```python
from build123d import *

# Parameters (mm, degrees)
BOSS_EXTRUDE2_DEPTH = 24.13
SKETCH3_W           = 24.13
SKETCH3_H           = 25.4
SKETCH3_R           = 8.89
CUT_EXTRUDE3_DEPTH  = 16.51
SKETCH4_W           = 138.37052371
SKETCH4_H           = 157.28988693
CUT_EXTRUDE4_DEPTH  = 8.89
CHAMFER1_SIZE       = 34.874144438
CHAMFER1_SIZE_2     = 10


with BuildPart() as part:
    # Sketch2 → Boss-Extrude2 (new body)
    # profile 1 of 2: a face of its own
    with BuildSketch(Plane(origin=(0, 0, 0), x_dir=(0, 0, -1), z_dir=(1, 0, 0))):
        Polygon((-111.06, -12.7), (-22.16, -12.7), (-22.16, 0), (-22.16, 12.7), (-111.06, 12.7), align=None)
    # profile 2 of 2: a face of its own
    with BuildSketch(Plane(origin=(0, 0, 0), x_dir=(0, 0, -1), z_dir=(1, 0, 0))):
        with BuildLine():
            Line((-22.16, -44.45), (-22.16, 44.45))
            ThreePointArc((-22.16, 44.45), (0, 66.61), (22.16, 44.45))
            Line((22.16, 44.45), (22.16, -44.45))
            ThreePointArc((22.16, -44.45), (0, -66.61), (-22.16, -44.45))
        make_face()
        with BuildLine():
            ThreePointArc((12, 44.45), (0, 56.45), (-12, 44.45))
            Line((-12, 44.45), (-12, -44.45))
            ThreePointArc((-12, -44.45), (0, -56.45), (12, -44.45))
            Line((12, -44.45), (12, 44.45))
        make_face(mode=Mode.SUBTRACT)
    extrude(amount=BOSS_EXTRUDE2_DEPTH)

    # Sketch3 → Cut-Extrude3 (cut)
    with BuildSketch(Plane.XY.offset(111.06)):
        with Locations((12.065, 0)):
            Rectangle(SKETCH3_W, SKETCH3_H)
        with Locations((10.4775, 0)):
            Circle(SKETCH3_R, mode=Mode.SUBTRACT)
    extrude(amount=-CUT_EXTRUDE3_DEPTH, mode=Mode.SUBTRACT)

    # Sketch4 → Cut-Extrude4 (cut)
    with BuildSketch(Plane.ZY):
        Rectangle(SKETCH4_W, SKETCH4_H)
    extrude(amount=-CUT_EXTRUDE4_DEPTH, mode=Mode.SUBTRACT)

    # Chamfer1
    # the kernel refuses this chamfer: 34.874144438, 10 mm, written as the material it adds along each edge
    with BuildSketch(Plane(origin=(8.89, 12.7, 69.185261855), x_dir=(0.010616657410321159, 0, -0.9999436417045873), z_dir=(0, -1, 0))) as chamfer1_piece_1_section:
        Polygon((CHAMFER1_SIZE * 0.999943641716, -CHAMFER1_SIZE * 0.0106166574104), (-CHAMFER1_SIZE_2 * 0.0106166574103, -CHAMFER1_SIZE_2 * 0.999943641705), (0, 0), align=None)
    chamfer1_piece_1 = extrude(amount=25.4, mode=Mode.PRIVATE)
    chamfer1_piece_1 = split(chamfer1_piece_1, bisect_by=Plane(origin=(0, 0, 56.832486902), z_dir=(1, 0, 0)), keep=Keep.TOP, mode=Mode.PRIVATE)
    add(chamfer1_piece_1)


solid = part.part
```
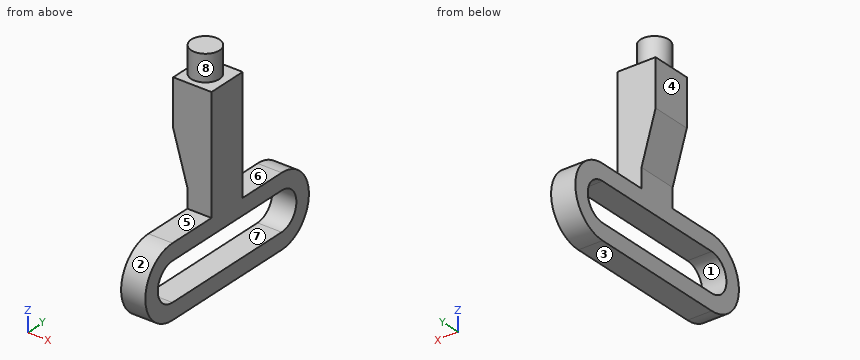
The listing builds one solid part. Answer for the finished solid, in the listing's coordinates (mm). Face numbers are marked on the shaded views. A direction names the side the tool comes from. Coordinates: 2 decimals unless noted, no trailing zeros. Write each loop counter-clockwise with the first axis right and the second up, starting at its lowest first coordinate (ties: lowest second). Pieces come first, ordered by that corner, then holes. Notation, with made-up numbers: (-3.75, 12.5) - (53.25, 12.5) arc R14 ccw to (53.25, 16.5) - close; hole circle Ø2 at (49.5, -33.75). An arc over 180 degrees is marked (long way). Return JSON: item names as keys, results as strings. Group by question number.
Q1. Flat-ended cylindrical pins translate along their axes: pin 1 Ø7 at (x, z) = (8.5, 41.5) entering from -Y; pin 2 Ø4 at (x, z) = (12, 66) entering from +Y; pin 3 Ø4.5 at (x, y) = (19.5, 19.5) entering from +Z; pin 4 Ø6 at (x, y) = (6.5, 28.5) entering from -Z. Find the tip coordinate at first contact, or state that the pin passes through.
Q2. Find the intervals of material crossed by line 1 along Z through (x, y) = (22.25, 9); line 2 along Z through (x, y) = (12.75, -25); line 3 along Y through (x, z) = (3, 73.5), in increasing order. Write a range as [from, to].
Q3. The part is cut by section C-C on x = 16.75. Write down the section's boundary in (y, z), and give its area (3 significant figures).
Q4. Which of the six approach directions +Z, -Z, +X, -X, +Y, -Y give full straight-line access (tool end or side, diameter ignored) to the marked faces 5, 6, 7 and 8?
Q5. The part is cut by section B-B on y = -38.5. Write down the section's boundary in (x, z), and give its area (3 significant figures).
Q6. The part is cut by section A-A on z = 0. Write down the section's boundary in (x, y), and give its area (3 significant figures).
Q7. The part is cut by section D-D on y = 0. Write down the section's boundary in (x, z), and give its area (3 significant figures).
Q8. For a pull along Z with two mould halves and no side action, classify the marked faces 1, 2, 3 and 4 as +Z half, -Z half, draft (parallel to the pull), parting line (faces both ways), or undercut.
Evaluation:
{
 "1": {"pin 1": "stops at y = -12.7", "pin 2": "stops at y = 12.7", "pin 3": "stops at z = 22.16", "pin 4": "stops at z = -22.16"},
 "2": {"line 1": "z = [-22.16, -12], [12, 94.55]", "line 2": "z = [-22.16, -12], [12, 22.16]", "line 3": "y = [-12.7, 12.7]"},
 "3": {"outline": "(-44.45, -22.16) - (44.45, -22.16) arc R22.16 ccw to (44.45, 22.16) - (12.7, 22.16) - (12.7, 94.55) - (6.3, 94.55) - (6.3, 111.06) - (-6.3, 111.06) - (-6.3, 94.55) - (-12.7, 94.55) - (-12.7, 22.16) - (-44.45, 22.16) arc R22.16 ccw to start; hole (-44.45, -12) - (44.45, -12) arc R12 ccw to (44.45, 12) - (-44.45, 12) arc R12 ccw to start", "area": "4,940 mm2"},
 "4": {"face 5": "+Z, +X, -X, -Y", "face 6": "+Z, +X, -X, +Y", "face 7": "+X, -X", "face 8": "+Z"},
 "5": {"outline": "(8.89, -22.16) - (24.13, -22.16) - (24.13, -12) - (8.89, -12) - close; (8.89, 12) - (24.13, 12) - (24.13, 22.16) - (8.89, 22.16) - close", "area": "310 mm2"},
 "6": {"outline": "(8.89, -66.61) - (24.13, -66.61) - (24.13, -56.45) - (8.89, -56.45) - close; (8.89, 56.45) - (24.13, 56.45) - (24.13, 66.61) - (8.89, 66.61) - close", "area": "310 mm2"},
 "7": {"outline": "(0, 65.31) - (8.89, 34.31) - (8.89, 12) - (24.13, 12) - (24.13, 94.55) - (19.37, 94.55) - (19.37, 111.06) - (1.59, 111.06) - (1.59, 94.55) - (0, 94.55) - close; (8.89, -22.16) - (24.13, -22.16) - (24.13, -12) - (8.89, -12) - close", "area": "2,100 mm2"},
 "8": {"face 1": "undercut", "face 2": "parting line", "face 3": "-Z half", "face 4": "draft"}
}
